Input: part model. Units: mm. Frame: model coordinates. Face numbers are marked on the shaded views. A direction names the side the tool comes from. Coordinates: 2 decimals unless noted, no trailing zeros. Write each loop counter-clockwise with the first axis right and the second up, starting at its lowest first coordinate (ties: lowest second). Pieces come first, ordered by that corner, then holes. Notation, with made-up numbers: (85.25, 9.5) - (109.25, 9.5) arc R16 ccw to (109.25, 37.5) - close; hole circle Ø8 at (74.25, -6.5). An arc over 180 degrees is marked (long way). Use CSV: the item, a comma, the result in double quotes.
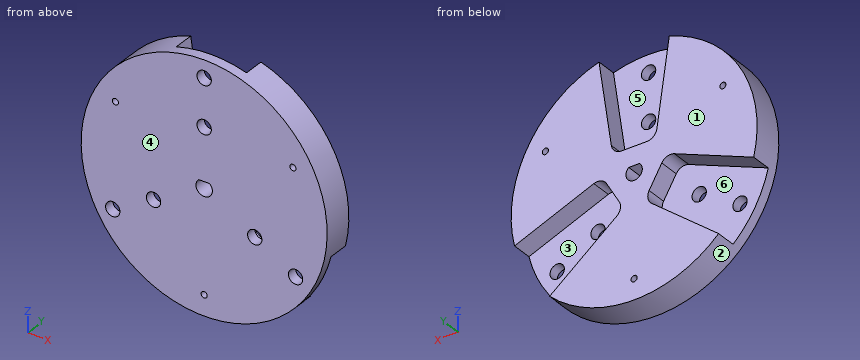
```python
from build123d import *

# Parameters (mm, degrees)
SKETCH1_R           = 60
BOSS_EXTRUDE1_DEPTH = 15
CUT_EXTRUDE1_REACH  = 88.168
CUT_EXTRUDE2_DEPTH  = 10
CUT_EXTRUDE3_REACH  = 87.44
SKETCH3_R           = 3.5
CIRPATTERN1_COUNT   = 3
CIRPATTERN2_COUNT   = 3
FILLET1_R           = 5
CUT_EXTRUDE4_REACH  = 88.168
SKETCH4_R           = 1.5
CIRPATTERN3_COUNT   = 3
BOSS_EXTRUDE2_REACH = 88.168


with BuildPart() as part:
    # Sketch1 → Boss-Extrude1 (new body)
    with BuildSketch(Plane(origin=(0, 0, 0), x_dir=(1, 0, 0), z_dir=(0, 1, 0))):
        with Locations(Location((0, 0, 0), (0, 0, 270))):
            Circle(SKETCH1_R)
    extrude(amount=BOSS_EXTRUDE1_DEPTH)

    # Sketch2 → Cut-Extrude1 (cut, up to next)
    with BuildSketch(Plane(origin=(0, 15, 0), x_dir=(1, 0, 0), z_dir=(0, 1, 0)), mode=Mode.PRIVATE) as cut_extrude1_sk1:
        with BuildLine():
            Line((-2.645751311, -3), (2.645751311, -3))
            ThreePointArc((2.645751311, -3), (0, 4), (-2.645751311, -3))
        make_face()
    cut_extrude1_tool1 = extrude(cut_extrude1_sk1.sketch, amount=-CUT_EXTRUDE1_REACH, mode=Mode.PRIVATE) & part.part
    add(cut_extrude1_tool1.solids().sort_by_distance((0, 15, -0.264732))[0], mode=Mode.SUBTRACT)

    # Sketch2_3 → Cut-Extrude2 (cut)
    with BuildSketch(Plane(origin=(0, 15, 0), x_dir=(1, 0, 0), z_dir=(0, 1, 0))):
        with BuildLine():
            Line((-2.645751311, -3), (2.645751311, -3))
            ThreePointArc((2.645751311, -3), (0, 4), (-2.645751311, -3))
        make_face()
        Polygon((-17.5, -60), (17.5, -60), (10.5, -12), (-10.5, -12), align=None)
    cut_extrude2 = extrude(amount=-CUT_EXTRUDE2_DEPTH, mode=Mode.SUBTRACT)

    # Sketch3 → Cut-Extrude3 (cut, up to next)
    with BuildSketch(Plane(origin=(0, 5, 0), x_dir=(1, 0, 0), z_dir=(0, 1, 0)), mode=Mode.PRIVATE) as cut_extrude3_sk1:
        with Locations(Location((0, -28.5, 0), (0, 0, 270))):
            Circle(SKETCH3_R)
    cut_extrude3_tool1 = extrude(cut_extrude3_sk1.sketch, amount=-CUT_EXTRUDE3_REACH, mode=Mode.PRIVATE) & part.part
    # Sketch3 → Cut-Extrude3 (cut, up to next)
    with BuildSketch(Plane(origin=(0, 5, 0), x_dir=(1, 0, 0), z_dir=(0, 1, 0)), mode=Mode.PRIVATE) as cut_extrude3_sk2:
        with Locations(Location((0, -51.5, 0), (0, 0, 270))):
            Circle(SKETCH3_R)
    cut_extrude3_tool2 = extrude(cut_extrude3_sk2.sketch, amount=-CUT_EXTRUDE3_REACH, mode=Mode.PRIVATE) & part.part
    cut_extrude3_1 = cut_extrude3_tool1.solids().sort_by_distance((0, 5, 28.5))[0]
    add(cut_extrude3_1, mode=Mode.SUBTRACT)
    cut_extrude3_2 = cut_extrude3_tool2.solids().sort_by_distance((0, 5, 51.5))[0]
    add(cut_extrude3_2, mode=Mode.SUBTRACT)
    cut_extrude3 = cut_extrude3_1 + cut_extrude3_2  # Cut-Extrude3 as one shape, for the pattern or mirror that repeats it

    # CirPattern1: Cut-Extrude2 ×3 about axis
    cirpattern1_axis = Axis((0, 0, 0), (0, 1, 0))
    for i in range(1, CIRPATTERN1_COUNT):
        add(cut_extrude2.rotate(cirpattern1_axis, i * 360 / CIRPATTERN1_COUNT), mode=Mode.SUBTRACT)

    # CirPattern2: Cut-Extrude3 ×3 about axis
    cirpattern2_axis = Axis((0, 0, 0), (0, 1, 0))
    for i in range(1, CIRPATTERN2_COUNT):
        add(cut_extrude3.rotate(cirpattern2_axis, i * 360 / CIRPATTERN2_COUNT), mode=Mode.SUBTRACT)

    # Fillet1
    fillet1_edges = [part.edges().sort_by_distance(p)[0] for p in [
        (10.5, 10, 12),
        (-10.5, 10, 12),
        (-15.642304845, 10, 3.09326674),
        (-5.142304845, 10, -15.09326674),
        (5.142304845, 10, -15.09326674),
        (15.642304845, 10, 3.09326674),
    ]]
    fillet(fillet1_edges, radius=FILLET1_R)

    # Sketch4 → Cut-Extrude4 (cut, up to next)
    with BuildSketch(Plane(origin=(0, 15, 0), x_dir=(1, 0, 0), z_dir=(0, 1, 0)), mode=Mode.PRIVATE) as cut_extrude4_sk1:
        with Locations(Location((0, 50, 0), (0, 0, 270))):
            Circle(SKETCH4_R)
    cut_extrude4_tool1 = extrude(cut_extrude4_sk1.sketch, amount=-CUT_EXTRUDE4_REACH, mode=Mode.PRIVATE) & part.part
    cut_extrude4 = cut_extrude4_tool1.solids().sort_by_distance((0, 15, -50))[0]
    add(cut_extrude4, mode=Mode.SUBTRACT)

    # CirPattern3: Cut-Extrude4 ×3 about axis
    cirpattern3_axis = Axis((0, 0, 0), (0, 1, 0))
    for i in range(1, CIRPATTERN3_COUNT):
        add(cut_extrude4.rotate(cirpattern3_axis, i * 360 / CIRPATTERN3_COUNT), mode=Mode.SUBTRACT)

    # Sketch5 → Boss-Extrude2 (add, up to next)
    with BuildSketch(Plane(origin=(0, 15, 0), x_dir=(1, 0, 0), z_dir=(0, 1, 0)), mode=Mode.PRIVATE) as boss_extrude2_sk1:
        with BuildLine():
            Line((-2.645751311, -3), (2.645751311, -3))
            ThreePointArc((2.645751311, -3), (0, -4), (-2.645751311, -3))
        make_face()
    boss_extrude2_tool1 = extrude(boss_extrude2_sk1.sketch, amount=-BOSS_EXTRUDE2_REACH, mode=Mode.PRIVATE) - part.part
    add(boss_extrude2_tool1.solids().sort_by_distance((0, 15, 3.404621))[0])


solid = part.part
```
(1) Cut plane D-D on x = -26. Return loops of the section in (y, z), and give its area (3 significant figures).
Check values:
outline,"(0, -54.07) - (15, -54.07) - (15, -31.56) - (5, -31.56) - (5, -17.49) - (0, -17.49) - close; (0, -11.01) - (5, -11.01) - (5, -1.03) - (15, -1.03) - (15, 54.07) - (0, 54.07) - close"
area,"1,280 mm^2"
(2) Ray query, probe 1 along X at (y, z) = (9, 25); probe 2 along X at (y, z) = (4, -25.75); probe 3 along Y at (x, z) = (7, 52). Return the intervals inside material, ascending. Write a range as from..to.
Check values:
probe 1,"-54.54..-44.8, -41.8..-12.4, 12.4..41.8, 44.8..54.54"
probe 2,"-54.19..-48.1, -41.1..41.1, 48.1..54.19"
probe 3,"0..5"
(3) Pin query (flat end, axial travel): pin 1 Ø9 at (x, z) = (-24.68, -14.25) entering from +Y; pin 2 Ø1 at (y, z) = (13.5, 6) entering from -X; pin 3 Ø3 at (x, y) = (-1.5, 11.5) entering from +Z; pin 4 Ø4 at (x, z) = (-44.6, -25.75) entering from -Y. Return the tip coordinate at first contact, or that it passes through.
Check values:
pin 1,"y = 5"
pin 2,"x = -59.75"
pin 3,"z = 12"
pin 4,"through"
(4) Cut plane B-B on z = 28.5. Return loops of the section in (x, y).
Check values:
outline,"(-52.8, 0) - (-3.5, 0) - (-3.5, 5) - (-12.91, 5) - (-12.91, 15) - (-52.8, 15) - close; (3.5, 0) - (52.8, 0) - (52.8, 15) - (12.91, 15) - (12.91, 5) - (3.5, 5) - close"
(5) Draft query along X for the marked faces 1, 2 and 3. Return one class per face: pulls with the +X half, pulls with the -X half, needs draft (parallel to the pull), parting line crosses it, or undercut.
Check values:
face 1,"needs draft"
face 2,"parting line crosses it"
face 3,"undercut"
(6) Cut plane A-A on x = 0. Return loops of the section in (y, z), and give its area (3 significant figures).
Check values:
outline,"(0, -60) - (15, -60) - (15, -51.5) - (0, -51.5) - close; (0, -48.5) - (15, -48.5) - (15, -4) - (0, -4) - close; (0, 3) - (15, 3) - (15, 12) - (5, 12) - (5, 25) - (0, 25) - close; (0, 32) - (5, 32) - (5, 48) - (0, 48) - close; (0, 55) - (5, 55) - (5, 60) - (0, 60) - close"
area,"1,100 mm^2"
(7) Reachability of the marked faces 4, 5 and 6 from +Z, -Z, +X, -X, +Y, -Y: full face, straight path, thin tool, end or side. Return the list, or none.
Check values:
face 4,"+Z, -Z, +X, -X, -Y"
face 5,"+Z, +Y"
face 6,"+Y"
(8) Cut plane C-C on y = 6.75. Return loops of the section in (x, z).
Check values:
outline,"(-58.37, -13.91) - (-19.66, 1.49) arc R5 cw to (-13.48, -0.65) - (-7.3, -11.35) arc R5 cw to (-8.54, -17.77) - (-41.23, -43.59) arc R60 ccw to (41.23, -43.59) - (8.54, -17.77) arc R5 cw to (7.3, -11.35) - (13.48, -0.65) arc R5 cw to (19.66, 1.49) - (58.37, -13.91) arc R60 ccw to (17.14, 57.5) - (11.12, 16.28) arc R5 cw to (6.18, 12) - (-6.18, 12) arc R5 cw to (-11.12, 16.28) - (-17.14, 57.5) arc R60 ccw to start; hole circle Ø3 at (-43.3, 25); hole (-2.65, 3) arc R4 ccw (long way) to (2.65, 3) - close; hole circle Ø3 at (0, -50); hole circle Ø3 at (43.3, 25)"
